from build123d import *

# Parameters (mm, degrees)
ESQUISSE1_R        = 1.5
ESQUISSE1_R_2      = 4.25
BOSS_EXTRU_1_DEPTH = 5
CONG_1_R           = 5


with BuildPart() as part:
    # Esquisse1 → Boss.-Extru.1 (new body)
    with BuildSketch(Plane.XY):
        Polygon((-20, 0), (20, 0), (20, 6), (15, 6), (15, 11), (20, 11), (20, 46), (15, 46), (15, 51), (20, 51), (20, 57), (-20, 57), (-25, 57), (-65, 57), (-65, 51), (-60, 51), (-60, 46), (-65, 46), (-65, 11), (-60, 11), (-60, 6), (-65, 6), (-65, 0), (-25, 0), align=None)
        with Locations((0, 48.5)):
            Circle(ESQUISSE1_R, mode=Mode.SUBTRACT)
        with Locations((0, 8.5)):
            Circle(ESQUISSE1_R, mode=Mode.SUBTRACT)
        with Locations((0, 28.5)):
            Circle(ESQUISSE1_R_2, mode=Mode.SUBTRACT)
        with Locations(Location((-45, 8.5, 0), (0, 0, 180))):
            Circle(ESQUISSE1_R, mode=Mode.SUBTRACT)
        with Locations(Location((-45, 28.5, 0), (0, 0, 180))):
            Circle(ESQUISSE1_R_2, mode=Mode.SUBTRACT)
        with Locations(Location((-45, 48.5, 0), (0, 0, 180))):
            Circle(ESQUISSE1_R, mode=Mode.SUBTRACT)
        Polygon((-20, 51), (-15, 51), (-15, 46), (-20, 46), (-25, 46), (-30, 46), (-30, 51), (-25, 51), align=None, mode=Mode.SUBTRACT)
        Polygon((-20, 11), (-15, 11), (-15, 6), (-20, 6), (-25, 6), (-30, 6), (-30, 11), (-25, 11), align=None, mode=Mode.SUBTRACT)
    extrude(amount=BOSS_EXTRU_1_DEPTH)

    # Congé1
    cong_1_edges = [part.edges().sort_by_distance(p)[0] for p in [
        (-65, 0, 2.5),
        (-65, 57, 2.5),
        (20, 57, 2.5),
        (20, 0, 2.5),
    ]]
    fillet(cong_1_edges, radius=CONG_1_R)


solid = part.part
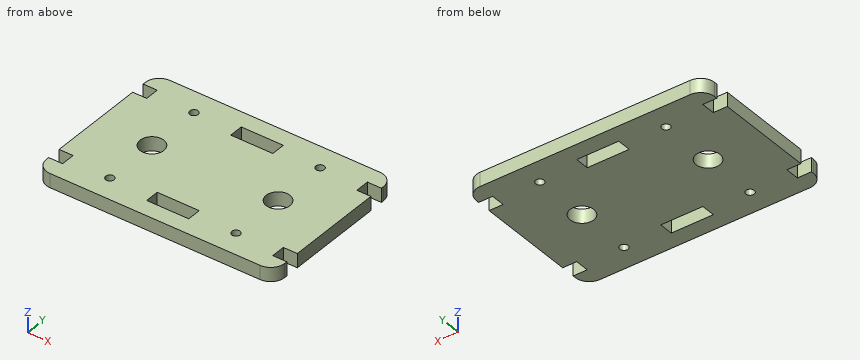
The model under review builds one solid part; all positions refer to its coordinate system, in mm. Give positions to 0.01 mm unless a question says otherwise; leave off trailing zeros. Order: outer loops, then holes, each group sorted by start corner. A loop starts at its lowest first (then second) coordinate and runs counter-clockwise, first axis right, second up. Notation, with made-up numbers: M -18.75,77 L 29.25,77 A23 cw 29.25,114 Z; hole C 8.25,80 d8. An arc over 180 degrees is marked long. One line per question, with ' | ' between items. Start each with the question number.
1) Consider section B-B, the plane x = -22. Give the boundary of the cut face in (y, z).
2) Consider section C-C, the plane x = -45. Give the boundary of the cut face in (y, z), then the cut area to 4 significant figures.
3) Clearance check with flat-ended pins moving along their axes: P1, Ø5, axis at x = -44, y = 47.5, coming from the -Z side; P2, Ø2.5, axis at x = -63, z = 1.5, coming from the +Y side; P3, Ø1.5, axis at y = 8.5, z = 2, coming from the +X side; P4, Ø2.5, axis at x = -62.5, z = 2, coming from the -Y side. State where each tip first meets the part, or that it passes through.
4) Wall thickness on L1, parallel to Y at x = -17.5, z = 2.8; L2, parallel to Y at x = 0, z = 1.3; L3, parallel to X at y = 32, z = 4.7: over which ranges is each line inside the solid? List them lowest first. Write a range as from..to.
5) Consider section A-A, the plane y = 28.5. Give the boundary of the cut face in (x, z).
6) Consider section D-D, the plane y = 48.5. Give the boundary of the cut face in (x, z), then the cut area to 3 significant figures.
Found:
1) outline: M 0,0 L 6,0 L 6,5 L 0,5 Z; M 11,0 L 46,0 L 46,5 L 11,5 Z; M 51,0 L 57,0 L 57,5 L 51,5 Z
2) outline: M 0,0 L 7,0 L 7,5 L 0,5 Z; M 10,0 L 24.25,0 L 24.25,5 L 10,5 Z; M 32.75,0 L 47,0 L 47,5 L 32.75,5 Z; M 50,0 L 57,0 L 57,5 L 50,5 Z | area: 212.5 mm²
3) P1: stops at z = 0 | P2: stops at y = 56.68 | P3: stops at x = 15 | P4: stops at y = 0.16
4) L1: y = 0..6, 11..46, 51..57 | L2: y = 0..7, 10..24.25, 32.75..47, 50..57 | L3: x = -65..-47.41, -42.59..-2.41, 2.41..20
5) outline: M -65,0 L -49.25,0 L -49.25,5 L -65,5 Z; M -40.75,0 L -4.25,0 L -4.25,5 L -40.75,5 Z; M 4.25,0 L 20,0 L 20,5 L 4.25,5 Z
6) outline: M -60,0 L -46.5,0 L -46.5,5 L -60,5 Z; M -43.5,0 L -30,0 L -30,5 L -43.5,5 Z; M -15,0 L -1.5,0 L -1.5,5 L -15,5 Z; M 1.5,0 L 15,0 L 15,5 L 1.5,5 Z | area: 270 mm²
